Autodesk Inventor part; units mm, degrees
ref_plane "YZ Plane" through (0, 0, 0) normal (1, 0, 0) x (0, 1, 0)
ref_plane "XZ Plane" through (0, 0, 0) normal (0, 1, 0) x (-1, 0, 0)
ref_plane "XY Plane" through (0, 0, 0) normal (0, 0, 1) x (1, 0, 0)
sketch "Sketch1" plane through (0, 0, 0) normal (0, 0, 1) x (1, 0, 0)
  line L0 (-39.5, 12) -> (39.5, 12)
  line L1 (39.5, 12) -> (39.5, -12)
  line L2 (39.5, -12) -> (-39.5, -12)
  line L3 (-39.5, -12) -> (-39.5, 12)
  line L4 (-39.5, 12) -> (39.5, -12) construction
  line L5 (39.5, 12) -> (-39.5, -12) construction
  point P0 (0, 0)
  dimension "d0" = 79
  dimension "d1" = 24
extrude "Extrusion1" add sketch "Sketch1" along normal blind 5.6
sketch "Sketch3" plane through (0, 0, 0) normal (0, 0, -1) x (-1, 0, 0)
  line L0 (-39.5, 12) -> (-31.5, 12)
  line L1 (-31.5, 12) -> (-31.5, 18.5)
  line L2 (-31.5, 18.5) -> (-39.5, 18.5)
  line L3 (-39.5, 18.5) -> (-39.5, 12)
  line L4 (-39.5, -12) -> (-31.5, -12)
  line L5 (-31.5, -12) -> (-31.5, -18.5)
  line L6 (-31.5, -18.5) -> (-39.5, -18.5)
  line L7 (-39.5, -18.5) -> (-39.5, -12)
  point P0 (0, 0)
  dimension "d8" = 8
  dimension "d9" = 6.5
  dimension "d10" = 6.5
extrude "Extrusion2" add sketch "Sketch3" against normal blind 38.6
chamfer "Chamfer1" distance 6.5 angle 45 2 edges at (31.5, -12, 2.8) (31.5, 12, 2.8)
sketch "Sketch5" plane through (0, 0, 0) normal (0, 0, -1) x (-1, 0, 0)
  line L0 (-25, -12) -> (39.5, -12)
  line L1 (39.5, 12) -> (-24.5, 12) construction
  line L2 (-24.5, 12) -> (-24.5, -12) construction
  line L3 (-24.5, -12) -> (39.5, -12) construction
  line L4 (39.5, -12) -> (39.5, 12) construction
  line L5 (-24.5, 12) -> (39.5, -12) construction
  line L6 (39.5, 12) -> (-24.5, -12) construction
  circle A0 centre (7.5, 0) radius 6.1
  line L7 (-17.5, 3) -> (32.5, 3) construction
  line L8 (32.5, 3) -> (32.5, -3) construction
  line L9 (32.5, -3) -> (-17.5, -3) construction
  line L10 (-17.5, -3) -> (-17.5, 3) construction
  line L11 (-17.5, 3) -> (32.5, -3) construction
  line L12 (32.5, 3) -> (-17.5, -3) construction
  circle A1 centre (-17.5, 0) radius 2.4
  circle A2 centre (32.5, 0) radius 2.4
  line L13 (1.4, 0) -> (1.4, -12)
  line L14 (13.6, 0) -> (13.6, -12)
  line L15 (13.6, -12) -> (1.4, -12)
  point P0 (0, 0)
  dimension "d29" = 64
  dimension "d30" = 12.2
  dimension "d31" = 50
  dimension "d32" = 4.8
  dimension "d33" = 4.8
extrude "Extrusion4" cut sketch "Sketch5" against normal blind 5.6
sketch "Sketch6" plane through (39.5, -18.5, 0) normal (1, 0, 0) x (0, 0, -1)
  line L0 (-38.6, 6.5) -> (-5.6, 6.5) construction
  line L1 (-5.6, 6.5) -> (-5.6, 1.5) construction
  line L2 (-5.6, 1.5) -> (-38.6, 1.5) construction
  line L3 (-38.6, 1.5) -> (-38.6, 6.5) construction
  line L4 (-38.6, 30.5) -> (-5.6, 30.5) construction
  line L5 (-5.6, 30.5) -> (-5.6, 35.5) construction
  line L6 (-5.6, 35.5) -> (-38.6, 35.5) construction
  line L7 (-38.6, 35.5) -> (-38.6, 30.5) construction
  line L8 (-38.6, 4) -> (-5.6, 4) construction
  line L9 (-38.6, 33) -> (-5.6, 33) construction
  line L10 (-38.6, 1.5) -> (-37.6, 1.5) construction
  line L11 (-37.6, 1.5) -> (-37.6, 6.5) construction
  line L12 (-37.6, 6.5) -> (-38.6, 6.5) construction
  line L13 (-38.6, 6.5) -> (-38.6, 1.5) construction
  line L14 (-37.6, 1.5) -> (-32.6, 1.5) construction
  line L15 (-32.6, 1.5) -> (-32.6, 6.5) construction
  line L16 (-32.6, 6.5) -> (-37.6, 6.5) construction
  line L17 (-37.6, 6.5) -> (-37.6, 1.5) construction
  line L18 (-38.6, 30.5) -> (-37.6, 30.5) construction
  line L19 (-37.6, 30.5) -> (-37.6, 35.5) construction
  line L20 (-37.6, 35.5) -> (-38.6, 35.5) construction
  line L21 (-38.6, 35.5) -> (-38.6, 30.5) construction
  line L22 (-37.6, 30.5) -> (-32.6, 30.5) construction
  line L23 (-32.6, 30.5) -> (-32.6, 35.5) construction
  line L24 (-32.6, 35.5) -> (-37.6, 35.5) construction
  line L25 (-37.6, 35.5) -> (-37.6, 30.5) construction
  line L26 (-37.6, 1.5) -> (-32.6, 6.5) construction
  line L27 (-37.6, 6.5) -> (-32.6, 1.5) construction
  line L28 (-37.6, 30.5) -> (-32.6, 35.5) construction
  line L29 (-37.6, 35.5) -> (-32.6, 30.5) construction
  line L30 (-38.6, 35.5) -> (-37.6, 35.5) construction
  line L31 (-37.6, 35.5) -> (-37.6, 30.5) construction
  line L32 (-37.6, 30.5) -> (-38.6, 30.5) construction
  line L33 (-38.6, 30.5) -> (-38.6, 35.5) construction
  line L34 (-5.6, 30.5) -> (-38.6, 30.5)
  line L35 (-32.6, 35.5) -> (-27.6, 35.5) construction
  line L36 (-27.6, 35.5) -> (-27.6, 30.5) construction
  line L37 (-27.6, 30.5) -> (-32.6, 30.5) construction
  line L38 (-32.6, 30.5) -> (-32.6, 35.5) construction
  line L39 (-27.6, 35.5) -> (-22.6, 35.5) construction
  line L40 (-22.6, 35.5) -> (-22.6, 30.5) construction
  line L41 (-22.6, 30.5) -> (-27.6, 30.5) construction
  line L42 (-27.6, 30.5) -> (-27.6, 35.5) construction
  line L43 (-32.6, 6.5) -> (-27.6, 6.5) construction
  line L44 (-27.6, 6.5) -> (-27.6, 1.5) construction
  line L45 (-27.6, 1.5) -> (-32.6, 1.5) construction
  line L46 (-32.6, 1.5) -> (-32.6, 6.5) construction
  line L47 (-27.6, 6.5) -> (-22.6, 6.5) construction
  line L48 (-22.6, 6.5) -> (-22.6, 1.5) construction
  line L49 (-22.6, 1.5) -> (-27.6, 1.5) construction
  line L50 (-27.6, 1.5) -> (-27.6, 6.5) construction
  line L51 (-22.6, 35.5) -> (-17.6, 35.5) construction
  line L52 (-17.6, 35.5) -> (-17.6, 30.5) construction
  line L53 (-17.6, 30.5) -> (-22.6, 30.5) construction
  line L54 (-22.6, 30.5) -> (-22.6, 35.5) construction
  line L55 (-22.6, 6.5) -> (-17.6, 6.5) construction
  line L56 (-17.6, 6.5) -> (-17.6, 1.5) construction
  line L57 (-17.6, 1.5) -> (-22.6, 1.5) construction
  line L58 (-22.6, 1.5) -> (-22.6, 6.5) construction
  line L59 (-17.6, 35.5) -> (-12.6, 35.5) construction
  line L60 (-12.6, 35.5) -> (-12.6, 30.5) construction
  line L61 (-12.6, 30.5) -> (-17.6, 30.5) construction
  line L62 (-17.6, 30.5) -> (-17.6, 35.5) construction
  line L63 (-17.6, 6.5) -> (-12.6, 6.5) construction
  line L64 (-12.6, 6.5) -> (-12.6, 1.5) construction
  line L65 (-12.6, 1.5) -> (-17.6, 1.5) construction
  line L66 (-17.6, 1.5) -> (-17.6, 6.5) construction
  line L67 (-32.6, 35.5) -> (-27.6, 30.5) construction
  line L68 (-27.6, 35.5) -> (-32.6, 30.5) construction
  line L69 (-27.6, 35.5) -> (-22.6, 30.5) construction
  line L70 (-27.6, 30.5) -> (-22.6, 35.5) construction
  line L71 (-22.6, 30.5) -> (-17.6, 35.5) construction
  line L72 (-22.6, 35.5) -> (-17.6, 30.5) construction
  line L73 (-17.6, 35.5) -> (-12.6, 30.5) construction
  line L74 (-12.6, 35.5) -> (-17.6, 30.5) construction
  line L75 (-17.6, 6.5) -> (-12.6, 1.5) construction
  line L76 (-12.6, 6.5) -> (-17.6, 1.5) construction
  line L77 (-22.6, 6.5) -> (-17.6, 1.5) construction
  line L78 (-17.6, 6.5) -> (-22.6, 1.5) construction
  line L79 (-27.6, 6.5) -> (-22.6, 1.5) construction
  line L80 (-22.6, 6.5) -> (-27.6, 1.5) construction
  line L81 (-32.6, 6.5) -> (-27.6, 1.5) construction
  line L82 (-27.6, 6.5) -> (-32.6, 1.5) construction
  point P0 (0, 18.5)
  point P1 (-35.1, 4)
  point P2 (-35.1, 33)
  point P3 (-30.1, 33)
  point P4 (-25.1, 33)
  point P5 (-20.1, 33)
  point P6 (-15.1, 33)
  point P7 (-15.1, 4)
  point P8 (-20.1, 4)
  point P9 (-25.1, 4)
  point P10 (-30.1, 4)
  dimension "d42" = 5
  dimension "d43" = 5
  dimension "d44" = 1
  dimension "d45" = 5
  dimension "d46" = 5
  dimension "d54" = 33
  dimension "d55" = 1
  dimension "d59" = 5
  dimension "d60" = 5
  dimension "d61" = 5
  dimension "d62" = 5
hole "Hole2" at (39.5, -14.5, 35.1) at (39.5, 14.5, 35.1) at (39.5, 14.5, 30.1) at (39.5, 14.5, 25.1) at (39.5, 14.5, 20.1) at (39.5, 14.5, 15.1) at (39.5, -14.5, 15.1) at (39.5, -14.5, 20.1) at (39.5, -14.5, 25.1) at (39.5, -14.5, 30.1) direction (-1, 0, 0) diameter 3 end through all
chamfer "Chamfer2" distance 6.4 angle 45 2 edges at (31.5, 15.25, 5.6) (31.5, -15.25, 5.6)
chamfer "Chamfer3" distance 5 angle 45 2 edges at (35.5, 12, 5.6) (35.5, -12, 5.6)
properties part number "Servo-Groove-Mount-E3D"
Build history of the part. All positions in model axes, mm. A direction names the side the tool comes from. Coordinates: 2 decimals unless noted, no trailing zeros. Write each loop counter-clockwise with the first axis right and the second up, starting at its lowest first coordinate (ties: lowest second). Pieces come first, ordered by that corner, then holes.
1. Drop flat-ended pins along their axis: pin 1 (7.5 mm diameter, centred on x = 3.5, y = 4, fed in from +Z); pin 2 (6 mm diameter, centred on x = -30, z = 3.5, fed in from -Y); pin 3 (1 mm diameter, centred on x = 6, z = 5, fed in from +Y). Give the stop position or say it passes through.
Answer block:
pin 1: stops at z = 5.6
pin 2: stops at y = -12
pin 3: stops at y = 12
2. Pull direction Y, two halves, no side cores. Call faces 4 (the flat face through (-8, 12, 3)), 5 (the cylindrical face through (35.4, -13.6, 16.3)), 6 (the flat face through (36, 15, 38.6)): released by +Y, released by -Y, zero draft, split by the parting line, or undercut.
Answer block:
face 4: released by +Y
face 5: undercut
face 6: zero draft
3. Band-saw the part on A-A, the plane z = 35.1. Give the cut face in (x, y), and give its area (3 significant figures).
Answer block:
outline: (31.5, -18.5) - (39.5, -18.5) - (39.5, -16) - (31.5, -16) - close; (31.5, -13) - (39.5, -13) - (39.5, -12) - (31.5, -12) - close; (31.5, 12) - (39.5, 12) - (39.5, 13) - (31.5, 13) - close; (31.5, 16) - (39.5, 16) - (39.5, 18.5) - (31.5, 18.5) - close
area: 56.0 mm2
4. Drill centre lines: probe 1 along Y at (x, z) = (34, 35); probe 2 along Y at (x, z) = (-32.5, 2.55); probe 3 along X at (y, z) = (-9, 4). Where is each one in solid material? Low to high.
Answer block:
probe 1: y = -18.5 to -16, -13 to -12, 12 to 13, 16 to 18.5
probe 2: y = -12 to -2.4, 2.4 to 12
probe 3: x = -39.5 to -13.6, -1.4 to 39.5
5. 3-axis set-ups, long thin cutter, end or side, ignore diameter. For faces 1 (the flat face through (34, -9.5, 8.1)), 2 (the flat face through (-13.6, -6, 3)), 3 (the flat face through (31.5, -15, 28)): which of +Z, -Z, +X, -X, +Y, -Y reach the whole face in a straight line?
Answer block:
face 1: +Z, +X, -X
face 2: +Z, -Z, -Y
face 3: +Z, -X, +Y, -Y
6. Band-saw the part on B-B, the plane x = -32.5. Give the cut face in (y, z).
Answer block:
outline: (-12, 0) - (-2.4, 0) - (-2.4, 5.6) - (-12, 5.6) - close; (2.4, 0) - (12, 0) - (12, 5.6) - (2.4, 5.6) - close
7. Band-saw the part on C-C, the plane y = -9. Give the cut face in (x, z), and give its area (3 significant figures).
Answer block:
outline: (-39.5, 0) - (-13.6, 0) - (-13.6, 5.6) - (-39.5, 5.6) - close; (-1.4, 0) - (39.5, 0) - (39.5, 7.6) - (27.1, 7.6) - (25.1, 5.6) - (-1.4, 5.6) - close
area: 401 mm2
